```python
from build123d import *

# Parameters (mm, degrees)
SKETCH1_W           = 140
SKETCH1_H           = 135
BOSS_EXTRUDE1_DEPTH = 1.2
CUT_EXTRUDE1_REACH  = 99.251
SKETCH2_R           = 2.75
SKETCH3_R           = 1.625
BOSS_EXTRUDE2_DEPTH = 7.5
SKETCH4_R           = 1.375
BOSS_EXTRUDE3_DEPTH = 7.5


with BuildPart() as part:
    # Sketch1 → Boss-Extrude1 (new body)
    with BuildSketch(Plane(origin=(0, 0, 0), x_dir=(1, 0, 0), z_dir=(0, 1, 0))):
        Rectangle(SKETCH1_W, SKETCH1_H)
    extrude(amount=BOSS_EXTRUDE1_DEPTH)

    # Sketch2 → Cut-Extrude1 (cut, up to next)
    with BuildSketch(Plane(origin=(0, 1.2, 0), x_dir=(1, 0, 0), z_dir=(0, 1, 0)), mode=Mode.PRIVATE) as cut_extrude1_sk1:
        with Locations(Location((65.75, -15.5, 0), (0, 0, 270))):
            Circle(SKETCH2_R)
    cut_extrude1_tool1 = extrude(cut_extrude1_sk1.sketch, amount=-CUT_EXTRUDE1_REACH, mode=Mode.PRIVATE) & part.part
    cut_extrude1 = cut_extrude1_tool1.solids().sort_by_distance((65.75, 1.2, 15.5))[0]
    add(cut_extrude1, mode=Mode.SUBTRACT)

    # Mirror1: Cut-Extrude1 across plane
    add(cut_extrude1.mirror(Plane(origin=(0, 0, 0), x_dir=(0, 0, 1), z_dir=(1, 0, 0))), mode=Mode.SUBTRACT)

    # Sketch3 → Boss-Extrude2 (add)
    with BuildSketch(Plane(origin=(0, 1.2, 0), x_dir=(1, 0, 0), z_dir=(0, 1, 0))):
        with Locations(Location((-60, 40, 0), (0, 0, 270))):
            Circle(SKETCH3_R)
        with Locations(Location((-60, 3, 0), (0, 0, 270))):
            Circle(SKETCH3_R)
    extrude(amount=BOSS_EXTRUDE2_DEPTH)

    # Sketch4 → Boss-Extrude3 (add)
    with BuildSketch(Plane(origin=(0, 1.2, 0), x_dir=(1, 0, 0), z_dir=(0, 1, 0))):
        with Locations(Location((56.5, -4.5, 0), (0, 0, 270))):
            Circle(SKETCH4_R)
        with Locations(Location((28.5, -4.5, 0), (0, 0, 270))):
            Circle(SKETCH4_R)
        with Locations(Location((23, 47, 0), (0, 0, 270))):
            Circle(SKETCH4_R)
    extrude(amount=BOSS_EXTRUDE3_DEPTH)


solid = part.part
```
Model file for the job. Use its own axes, mm. A direction names the side the tool comes from. Round coordinates to 2 decimals unless told otherwise and drop trailing zeros. Order: outer loops, then holes, each group sorted by start corner. A loop starts at its lowest first (then second) coordinate and runs counter-clockwise, first axis right, second up. Notation, with made-up numbers: M 30,89 L 48,89 A18 cw 48,110 Z; hole C 34,-12 d5. An arc over 180 degrees is marked long. Use CSV: the item, a comma, the result in double quotes.
Item 1: Pull direction Z, two halves, no side cores. Call faces 3 (the face through (68.477, 0.608, 15.142)), 4 (the face through (-1, 0, -1)): released by +Z, released by -Z, zero draft, split by the parting line, or undercut.
Worked answers:
face 3,"undercut"
face 4,"zero draft"
Item 2: Pin check, flat tips, straight feed: pin 1 (5 mm diameter, centred on x = -42.5, z = 41.5, fed in from +Y); pin 2 (5 mm diameter, centred on y = 7, z = -39, fed in from -X) (3 decimals). Stop position of each tip, or through.
Worked answers:
pin 1,"y = 1.2"
pin 2,"x = -61.625"
Item 3: Saw through at C-C (y = 4). List the corners of the cut face in (x, z) (3 decimals).
Worked answers:
outline,"C -60,-40 d3.25; C -60,-3 d3.25; C 23,-47 d2.75; C 28.5,4.5 d2.75; C 56.5,4.5 d2.75"
Item 4: Probe probe 1 along X at (y, z) = (0.6, 15.5); probe 2 along Z at (x, y) = (-65.75, 0.7); probe 3 along Y at (x, z) = (47.5, 44). List the from-to ranges inside material, lowest first.
Worked answers:
probe 1,"-70 to -68.5, -63 to 63, 68.5 to 70"
probe 2,"-67.5 to 12.75, 18.25 to 67.5"
probe 3,"0 to 1.2"
Item 5: Saw through at D-D (x = -60). List the corners of the cut face in (y, z) (3 decimals), plus the area to 3 significant figures.
Worked answers:
outline,"M 0,-67.5 L 1.2,-67.5 L 1.2,-41.625 L 8.7,-41.625 L 8.7,-38.375 L 1.2,-38.375 L 1.2,-4.625 L 8.7,-4.625 L 8.7,-1.375 L 1.2,-1.375 L 1.2,67.5 L 0,67.5 Z"
area,"211 mm²"
Item 6: Saw through at A-A (x = 65.75). List the corners of the cut face in (y, z).
Worked answers:
outline,"M 0,-67.5 L 1.2,-67.5 L 1.2,12.75 L 0,12.75 Z; M 0,18.25 L 1.2,18.25 L 1.2,67.5 L 0,67.5 Z"
Item 7: Saw through at B-B (z = -3). List the corners of the cut face in (x, y) (3 decimals), plus the area to 3 significant figures.
Worked answers:
outline,"M -70,0 L 70,0 L 70,1.2 L -58.375,1.2 L -58.375,8.7 L -61.625,8.7 L -61.625,1.2 L -70,1.2 Z"
area,"192 mm²"
Item 8: Which spindle directions (+Z, -Z, +X, -X, +Y, -Y) get a long thin tool onto all of the face, cutting with end or side? Do faces 1 (the face through (-61.586, 4.898, -3.352)), 2 (the face through (-68.477, 0.608, 15.142)). Say none if no direction does.
Worked answers:
face 1,"+Y"
face 2,"+Y, -Y"
